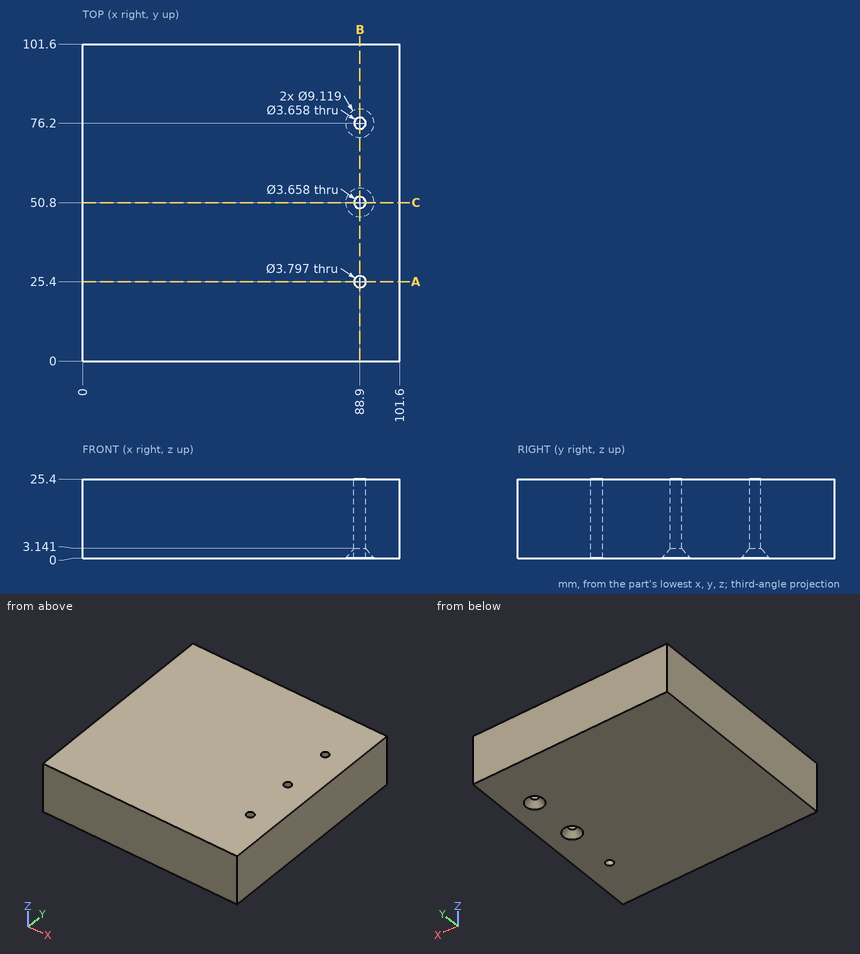
Input: dimensioned drawing with shaded views. Units: mm. Origin: part minimum x, y, z. Give positions to 0.01 mm unless a question says otherwise; leave off trailing zeros. Write each loop counter-clockwise with the first axis right and the second up, starting at its lowest first coordinate (ties: lowest second). Pieces come first, ordered by that corner, then holes.
Q1. Section C-C, the plane y = 50.8. Output: boundary loops of the cut face in (x, z).
Q2. Material intervals for probe 1 along Y at (x, z) = (88.9, 19.5); probe 2 along X at (y, z) = (25.4, 13.25); probe 3 along X at (y, z) = (50.8, 17.5), sorted ascending.
Q3. Section B-B, the plane x = 88.9. Output: boundary loops of the cut face in (y, z).
Q4. First-contact query: P1, Ø8, axis at y = 66, z = 8.5, coming from the -X side. Flat tip, straight axial feed; report the tip coordinate or a pass-through.
Q5. Section A-A, the plane y = 25.4. Output: boundary loops of the cut face in (x, z).
Filled in:
1. outline: (0, 0) - (84.34, 0) - (87.07, 3.14) - (87.07, 25.4) - (0, 25.4) - close; (90.73, 3.14) - (93.46, 0) - (101.6, 0) - (101.6, 25.4) - (90.73, 25.4) - close
2. probe 1: y = 0 to 23.5, 27.3 to 48.97, 52.63 to 74.37, 78.03 to 101.6
2. probe 2: x = 0 to 87, 90.8 to 101.6
2. probe 3: x = 0 to 87.07, 90.73 to 101.6
3. outline: (0, 0) - (23.5, 0) - (23.5, 25.4) - (0, 25.4) - close; (27.3, 0) - (46.24, 0) - (48.97, 3.14) - (48.97, 25.4) - (27.3, 25.4) - close; (52.63, 3.14) - (55.36, 0) - (71.64, 0) - (74.37, 3.14) - (74.37, 25.4) - (52.63, 25.4) - close; (78.03, 3.14) - (80.76, 0) - (101.6, 0) - (101.6, 25.4) - (78.03, 25.4) - close
4. P1: stops at x = 0
5. outline: (0, 0) - (87, 0) - (87, 25.4) - (0, 25.4) - close; (90.8, 0) - (101.6, 0) - (101.6, 25.4) - (90.8, 25.4) - close
